Source: CAD feature listing. Evaluate the final solid. Frame: model axes, mm. Face numbers are marked on the shaded views. A direction names the side the tool comes from. Coordinates: 2 decimals unless noted, no trailing zeros. Write each loop counter-clockwise with the first axis right and the second up, starting at its lowest first coordinate (ties: lowest second). Pieces come first, ordered by that corner, then holes. Notation, with made-up numbers: M 87.25,40.25 L 144.25,40.25 A10 cw 144.25,55.25 Z; hole C 4,-29.5 d8. An arc over 180 degrees is marked long. Answer as CSV lines item,"result". Start each with the question number.
1. Line query: probe 1 along Y at (x, z) = (0, 9.25) (3 decimals); probe 2 along Z at (x, y) = (-55, 2); probe 3 along Y at (x, z) = (-53.5, -9). Output: solid intervals per line, ascending. Write a range as [from, to].
2. Section B-B on x = 0. Return the cut outline in (y, z) (3 decimals), plus the area to 3 significant figures.
3. Section A-A on y = 38.1. Return the cut outline in (x, z) (3 decimals).
4. Section C-C on y = -57. Return the cut outline in (x, z).
5. Mould query, pull axis Y, two halves, no side actions, for the marked faces 1, 2 and 3. Classes: pulls with the +Y half, pulls with the -Y half, needs draft (parallel to the pull), parting line crosses it, or undercut.
6. Reachability of the marked faces 4, 5, 6, 7 and 8 from +Z, -Z, +X, -X, +Y, -Y: full face, straight path, thin tool, end or side. Return the list, or none.
7. Contact query for flat-ended pins moving along their axis: pin 1 Ø1.9 at (x, z) = (53.5, 9.5) entering from -Y; pin 2 Ø13.5 at (x, z) = (-28.5, -7.5) entering from +Y; pin 3 Ø4 at (x, z) = (-23, -7.5) entering from -Y; pin 4 Ø2 at (x, y) = (-4.5, -75) entering from -Z. Output: stop coordinate, or through.
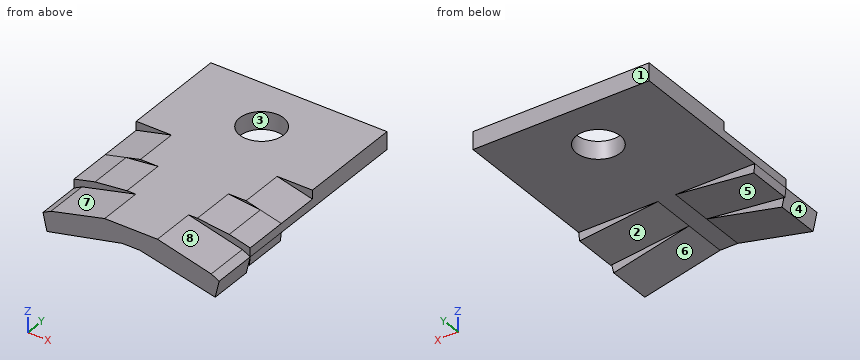
```python
from build123d import *

# Parameters (mm, degrees)
F0_W     = 127
F0_H     = 76.2
F0_R     = 15.875
F1_DEPTH = 12.7
F3_DEPTH = 31.75
F5_START = 31.75
F5_DEPTH = 31.75
F7_START = 63.5
F7_DEPTH = 31.75


with BuildPart() as f1:
    # F0 (on Top) → F1 (new body)
    with BuildSketch(Plane.XY):
        with Locations((0, 38.1)):
            Rectangle(F0_W, F0_H)
        with Locations((0, 38.1)):
            Circle(F0_R, mode=Mode.SUBTRACT)
    extrude(amount=F1_DEPTH)

    # F2 (on Front) → F3 (join)
    with BuildSketch(Plane.XZ):
        Polygon((-6.35, 0), (0, 0), (6.35, 0), (63.5, 0), (63.5, 6.35), (38.1, 12.7), (-38.1, 12.7), (-63.5, 6.35), (-63.5, 0), align=None)
    extrude(amount=F3_DEPTH)

    # F4 (on Front) → F5 (join)
    with BuildSketch(Plane.XZ.offset(F5_START)):
        Polygon((-6.35, 0), (0, 0), (6.35, 0), (62.7944444444, -6.3106807365), (63.5, 0), (63.5, 6.35), (48.3745158286, 10.1313710429), (25.4, 12.7), (-25.4, 12.7), (-48.3745158286, 10.1313710429), (-63.5, 6.35), (-63.5, 0), (-62.7944444444, -6.3106807365), align=None)
    extrude(amount=F5_DEPTH)

    # F6 (on Front) → F7 (join)
    with BuildSketch(Plane.XZ.offset(F7_START)):
        Polygon((-6.35, 0), (0, 0), (6.35, 0), (60.6777777778, -12.3824497467), (63.5, 0), (57.7921046631, 3.0144738342), (19.05, 12.7), (-19.05, 12.7), (-57.7921046631, 3.0144738342), (-63.5, 0), (-60.6777777778, -12.3824497467), align=None)
    extrude(amount=F7_DEPTH)


solid = f1.part
```
Values:
1,probe 1,"[-95.25, 22.225], [53.975, 76.2]"
1,probe 2,"[0, 12.7]"
1,probe 3,"[-95.25, -63.5]"
2,outline,"M -95.25,0 L 22.225,0 L 22.225,12.7 L -95.25,12.7 Z; M 53.975,0 L 76.2,0 L 76.2,12.7 L 53.975,12.7 Z"
2,area,"1,770 mm²"
3,outline,"M -63.5,0 L -15.875,0 L -15.875,12.7 L -63.5,12.7 Z; M 15.875,0 L 63.5,0 L 63.5,12.7 L 15.875,12.7 Z"
4,outline,"M -63.5,0 L -62.79,-6.31 L -6.35,0 L 6.35,0 L 62.79,-6.31 L 63.5,0 L 63.5,6.35 L 48.37,10.13 L 25.4,12.7 L -25.4,12.7 L -48.37,10.13 L -63.5,6.35 Z"
5,face 1,"pulls with the +Y half"
5,face 2,"needs draft"
5,face 3,"undercut"
6,face 4,"-Z, -X, -Y"
6,face 5,"-Z, +Y"
6,face 6,"-Z, +Y, -Y"
6,face 7,"+Z, -X, -Y"
6,face 8,"+Z, +X, -Y"
7,pin 1,"y = -63.5"
7,pin 2,"y = -31.75"
7,pin 3,"through"
7,pin 4,"z = 0"
